from build123d import *

# Parameters (mm, degrees)
SKETCH1_W           = 15
SKETCH1_H           = 10
BOSS_EXTRUDE1_DEPTH = 2
SKETCH2_W           = 2
SKETCH2_H           = 10
BOSS_EXTRUDE2_DEPTH = 8
SKETCH3_R           = 2.5
CUT_EXTRUDE1_DEPTH  = 19.708286934
SKETCH4_R           = 0.8
CUT_EXTRUDE2_DEPTH  = 13.051970793


with BuildPart() as part:
    # Sketch1 → Boss-Extrude1 (new body)
    with BuildSketch(Plane.XY):
        Rectangle(SKETCH1_W, SKETCH1_H)
    extrude(amount=BOSS_EXTRUDE1_DEPTH)

    # Sketch2 → Boss-Extrude2 (add)
    with BuildSketch(Plane.XY.offset(2)):
        with Locations((-6.5, 0)):
            Rectangle(SKETCH2_W, SKETCH2_H)
        with Locations((6.5, 0)):
            Rectangle(SKETCH2_W, SKETCH2_H)
    extrude(amount=BOSS_EXTRUDE2_DEPTH)

    # Sketch3 → Cut-Extrude1 (cut, through all)
    with BuildSketch(Plane.ZY.offset(7.5)):
        with Locations(Location((6, 0, 0), (0, 0, 270))):
            Circle(SKETCH3_R)
    extrude(amount=-CUT_EXTRUDE1_DEPTH, mode=Mode.SUBTRACT)

    # Sketch4 → Cut-Extrude2 (cut, through all)
    with BuildSketch(Plane.XY.offset(2)):
        Circle(SKETCH4_R)
    extrude(amount=-CUT_EXTRUDE2_DEPTH, mode=Mode.SUBTRACT)


solid = part.part
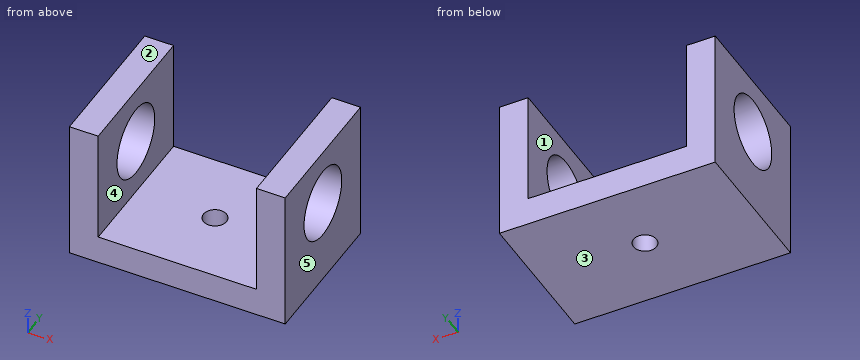
Geometry check sheet. Reference: the model listing, model coordinates, mm. Face numbers are marked on the shaded views. A direction names the side the tool comes from. Round coordinates to 2 decimals unless told otherwise and drop trailing zeros. Order: outer loops, then holes, each group sorted by start corner. A loop starts at its lowest first (then second) coordinate and runs counter-clockwise, first axis right, second up. Notation, with made-up numbers: M 28.25,-13.75 L 70.25,-13.75 A12 ccw 70.25,3.25 Z; hole C 78,8 d7. An arc over 180 degrees is marked long. Answer in a Markdown table with one row per item.
(1) Draft check along X on the marked faces 3, 4 and 5. Enter one of: released by +X, released by -X, zero draft, split by the parting line, or undercut.
Responses:
| item | result |
|---|---|
| face 3 | zero draft |
| face 4 | undercut |
| face 5 | released by +X |
(2) Tool access check on the marked faces 1 and 2. Record the directions out of +Z, -Z, +X, -X, +Y, -Y that give a thin tool (end or side, any length) a straight path to the whole face; none if there is none.
Responses:
| item | result |
|---|---|
| face 1 | +Z, +Y, -Y |
| face 2 | +Z, +X, -X, +Y, -Y |
(3) Scan lines: probe 1 along X at (y, z) = (2.5, 4.75); probe 2 along Y at (x, z) = (0, 1.4); probe 3 along Z at (x, y) = (-6.85, 0). Record each from-to range of solid material in increasing order. Write a range as from..to.
Responses:
| item | result |
|---|---|
| probe 1 | x = -7.5..-5.5, 5.5..7.5 |
| probe 2 | y = -5..-0.8, 0.8..5 |
| probe 3 | z = 0..3.5, 8.5..10 |
(4) Sectioned sample at C-C, the plane z = 6. Record the cut outline in (x, y).
Responses:
| item | result |
|---|---|
| outline | M -7.5,-5 L -5.5,-5 L -5.5,-2.5 L -7.5,-2.5 Z; M -7.5,2.5 L -5.5,2.5 L -5.5,5 L -7.5,5 Z; M 5.5,-5 L 7.5,-5 L 7.5,-2.5 L 5.5,-2.5 Z; M 5.5,2.5 L 7.5,2.5 L 7.5,5 L 5.5,5 Z |
(5) Sectioned sample at D-D, the plane y = 0. Record the cut outline in (x, z).
Responses:
| item | result |
|---|---|
| outline | M -7.5,0 L -0.8,0 L -0.8,2 L -5.5,2 L -5.5,3.5 L -7.5,3.5 Z; M -7.5,8.5 L -5.5,8.5 L -5.5,10 L -7.5,10 Z; M 0.8,0 L 7.5,0 L 7.5,3.5 L 5.5,3.5 L 5.5,2 L 0.8,2 Z; M 5.5,8.5 L 7.5,8.5 L 7.5,10 L 5.5,10 Z |
(6) Go/stop test with a flat-tipped pin: P1, Ø2, axis at x = -3, z = 7.5, coming from the -Y side. Record where the tip stops, or that it passes through.
Responses:
| item | result |
|---|---|
| P1 | passes through |
(7) Sectioned sample at A-A, the plane x = 0. Record the cut outline in (y, z).
Responses:
| item | result |
|---|---|
| outline | M -5,0 L -0.8,0 L -0.8,2 L -5,2 Z; M 0.8,0 L 5,0 L 5,2 L 0.8,2 Z |
(8) Sectioned sample at B-B, the plane z = 8.75. Record the cut outline in (x, y).
Responses:
| item | result |
|---|---|
| outline | M -7.5,-5 L -5.5,-5 L -5.5,5 L -7.5,5 Z; M 5.5,-5 L 7.5,-5 L 7.5,5 L 5.5,5 Z |
